```python
from build123d import *

# Parameters (mm, degrees)
CONE001_W         = 10
CONE001_H         = 10
FILLET002_R       = 3
BOX007_W          = 10.4
BOX007_H          = 5.2
BOX007_DEPTH      = 5.2
BOX008_W          = 40
BOX008_H          = 10
BOX008_DEPTH      = 3
CYLINDER011_R     = 5.2
CYLINDER011_DEPTH = 10


with BuildPart() as part:
    # Cone001 → Cone001 (revolve)
    with BuildSketch(Plane.XZ):
        with Locations((5, 5)):
            Rectangle(CONE001_W, CONE001_H)
    revolve(axis=Axis((0, 0, 0), (0, 0, 1)))

    # Fillet002
    fillet002_edges = [part.edges().sort_by_distance(p)[0] for p in [
        (-10, 0, 0),
    ]]
    fillet(fillet002_edges, radius=FILLET002_R)

    # Box007 → Box007 (cut)
    with BuildSketch(Plane(origin=(-5.2, -5.2, 0), x_dir=(1, 0, 0), z_dir=(0, 0, 1))):
        with Locations((5.2, 2.6)):
            Rectangle(BOX007_W, BOX007_H)
    extrude(amount=BOX007_DEPTH, mode=Mode.SUBTRACT)

    # Box008 → Box008 (join)
    with BuildSketch(Plane(origin=(-20, -5, 7), x_dir=(1, 0, 0), z_dir=(0, 0, 1))):
        with Locations((20, 5)):
            Rectangle(BOX008_W, BOX008_H)
    extrude(amount=BOX008_DEPTH)

    # Cylinder011 → Cylinder011 (cut)
    with BuildSketch(Plane.XY):
        Circle(CYLINDER011_R)
    extrude(amount=CYLINDER011_DEPTH, mode=Mode.SUBTRACT)


with BuildPart() as part_1:
    # Body006 placement: moved
    add(part.part.moved(Location((1, -43, -10))))


solid = part_1.part
```
Design review of the part built by this model. Coordinates are the model's own, in mm. A direction names the side the tool comes from. Give positions to 0.01 mm unless a question says otherwise; leave off trailing zeros. Order: outer loops, then holes, each group sorted by start corner. A loop starts at its lowest first (then second) coordinate and runs counter-clockwise, first axis right, second up. Notation, with made-up numbers: (-8, 46) - (29, 46) arc R28 ccw to (29, 77) - close; hole circle Ø4 at (19.25, 78.25). An arc over 180 degrees is marked (long way). Use a Markdown table: item, result. Add a question column.
(1) Add section B-B on z = -8.75. Give the boundary of the cut face in (x, y), then the cut area to 3 significant figures.
(2) Clearance check with flat-ended pins moving along their axes: P1, Ø0.9, axis at x = 16.5, z = -1, coming from the +Y side; P2, Ø3, axis at x = -13, y = -43.5, coming from the -Z side; P3, Ø4, axis at y = -46.5, z = -7, coming from the +X side; P4, Ø1.6, axis at x = -1, y = -44.5, coming from the -Z side. State where each tip first meets the part, or that it passes through.
(3) Mouldability with a two-part tool opening along X and no side actions: class faces 4 (the face through (-4, -41, 0)), 5 (the face through (-4.2, -46, -7)), 6 (the face through (-8.99, -42.56, -3.45)), 7 (the face through (-3, -47, -4.8)) as +X half, -X half, draft (parallel to the pull), parting line (faces both ways), or undercut.
(4) Add section A-A on z = -4. Give the boundary of the cut face in (x, y), then the cut area to 3 significant figures.
(5) Wall thickness on probe 1 along Y at (x, z) = (1, -4); probe 2 along X at (y, z) = (-43, -2.5); probe 3 along X at (y, z) = (-43, -4.5): over which ranges is each line inside the solid? List them lowest first. Write a range as [from, to].
(6) Machinability: for faces 1 (the face through (15, -48, -2)), 2 (the face through (5, -47, -4.8)), 3 (the face through (-13, -48, -2)), which of the approach directions +Z, -Z, +X, -X, +Y, -Y give a long, thin tool a straight path to every point of the face, cutting with its end or side? Answer none if there is none.
Report:
| question | item | result |
|---|---|---|
| 1 | outline | circle Ø18.87 at (1, -43); hole (-4.2, -48.2) - (6.2, -48.2) - (6.2, -43) arc R5.2 ccw to (-4.2, -43) - close |
| 1 | area | 183 mm² |
| 2 | P1 | stops at y = -38 |
| 2 | P2 | stops at z = -3 |
| 2 | P3 | stops at x = 10.89 |
| 2 | P4 | passes through |
| 3 | face 4 | draft |
| 3 | face 5 | undercut |
| 3 | face 6 | parting line |
| 3 | face 7 | undercut |
| 4 | outline | circle Ø20 at (1, -43); hole circle Ø10.4 at (1, -43) |
| 4 | area | 229 mm² |
| 5 | probe 1 | y = [-53, -48.2], [-37.8, -33] |
| 5 | probe 2 | x = [-19, -4.2], [6.2, 21] |
| 5 | probe 3 | x = [-9, -4.2], [6.2, 11] |
| 6 | face 1 | +Z, -Z, +X, -Y |
| 6 | face 2 | -Z |
| 6 | face 3 | +Z, -Z, -X, -Y |
